```python
from build123d import *

# Parameters (mm, degrees)
F0_W     = 5
F0_H     = 40
F1_DEPTH = 5
F0_R     = 12.5
F2_DEPTH = 12
F0_R_2   = 5
F3_DEPTH = 5
F4_R     = 6
F5_DEPTH = 5
F6_R     = 6
F7_DEPTH = 5


with BuildPart() as f1:
    # F0 (on Top) → F1 (new body)
    with BuildSketch(Plane.XY):
        with Locations((37.5, 0)):
            Rectangle(F0_W, F0_H)
        with BuildLine():
            Line((0, -20), (35, -20))
            Line((35, -20), (35, 20))
            Line((35, 20), (0, 20))
            ThreePointArc((0, 20), (14.142136, 14.142136), (20, 0))
            ThreePointArc((20, 0), (14.142136, -14.142136), (0, -20))
        make_face()
        with BuildLine():
            Line((-35, -20), (0, -20))
            ThreePointArc((0, -20), (-20, 0), (0, 20))
            Line((0, 20), (-35, 20))
            Line((-35, 20), (-35, -20))
        make_face()
        with Locations((-37.5, 0)):
            Rectangle(F0_W, F0_H)
    extrude(amount=F1_DEPTH)

    # F0 (on Top) → F2 (join)
    with BuildSketch(Plane.XY):
        with BuildLine():
            ThreePointArc((0, 20), (-20, 0), (0, -20))
            ThreePointArc((0, -20), (14.142136, -14.142136), (20, 0))
            ThreePointArc((20, 0), (14.142136, 14.142136), (0, 20))
        make_face()
        Circle(F0_R, mode=Mode.SUBTRACT)
    extrude(amount=F2_DEPTH)

    # F0 (on Top) → F3 (join)
    with BuildSketch(Plane.XY):
        Circle(F0_R)
        Circle(F0_R_2, mode=Mode.SUBTRACT)
    extrude(amount=F3_DEPTH)

    # F4 (on face) → F5 (join)
    with BuildSketch(Plane(origin=(-40, 0, 0), x_dir=(0, -1, 0), z_dir=(-1, 0, 0))):
        with BuildLine():
            Line((20, 0), (-20, 0))
            Line((-20, 0), (-20, -37))
            ThreePointArc((-20, -37), (0, -57), (20, -37))
            Line((20, -37), (20, 0))
        make_face()
        with Locations((0, -37)):
            Circle(F4_R, mode=Mode.SUBTRACT)
    extrude(amount=-F5_DEPTH)

    # F6 (on face) → F7 (join)
    with BuildSketch(Plane.YZ.offset(40)):
        with BuildLine():
            Line((-20, 5), (-20, 0))
            Line((-20, 0), (-20, -37))
            ThreePointArc((-20, -37), (0, -57), (20, -37))
            Line((20, -37), (20, 0))
            Line((20, 0), (20, 5))
            Line((20, 5), (-20, 5))
        make_face()
        with Locations((0, -37)):
            Circle(F6_R, mode=Mode.SUBTRACT)
    extrude(amount=-F7_DEPTH)


solid = f1.part
```
CAD build for the part. Positions are in the model's coordinates, mm. A direction names the side the tool comes from. Coordinates: 2 decimals unless noted, no trailing zeros. Order: outer loops, then holes, each group sorted by start corner. A loop starts at its lowest first (then second) coordinate and runs counter-clockwise, first axis right, second up. Notation, with made-up numbers: (6, 58) -> (65, 58) arc R33 cw to (65, 89) -> close; hole circle Ø5 at (35.5, -16). An arc over 180 degrees is marked (long way). Use one line per item in the form item = value. Start each with the question number.
1) Band-saw the part on B-B on z = -36. Give the cut face in (x, y).
2) Band-saw the part on A-A on z = -24. Give the cut face in (x, y), then the cut area to 3 significant figures.
3) Drop flat-ended pins along their axis: pin 1 (20 mm diameter, centred on x = -9, y = -6, fed in from -Z); pin 2 (20 mm diameter, centred on x = 0, y = 0, fed in from +Z). Give the stop position or say it passes through.
4) Tool access for faces 1 (the cylindrical face through (11.923, 3.755, 8.451)), 2 (the flat face through (7, 0, 0)), 3 (the flat face through (29, 0, 5)): list every direction of +Z, -Z, +X, -X, +Y, -Y with a clear straight run to the whole face (end or side of a thin tool).
5) Drill centre lines: L1, parallel to X at y = 11, z = -2; L2, parallel to Y at x = 0, z = 7.5; L3, parallel to Y at x = 0, z = 2.5. Where is each one in solid material? Low to high. Write a range as [from, to].
6) Band-saw the part on C-C on x = -25. Give the cut face in (y, z), then the cut area to 3 significant figures.
7) Band-saw the part on D-D on y = -14.5. Give the cut face in (x, z).
8) Pull direction X, two halves, no side cores. Call faces 4 (the flat face through (40, 0, -26)), 5 (the flat face through (35, 0, -28)), 6 (the cylindrical face through (-37.535, 1.301, -42.857)): +X half, -X half, draft (parallel to the pull), parting line (faces both ways), or undercut.
Entries:
q1.outline = (-40, -20) -> (-35, -20) -> (-35, -5.92) -> (-40, -5.92) -> close; (-40, 5.92) -> (-35, 5.92) -> (-35, 20) -> (-40, 20) -> close; (35, -20) -> (40, -20) -> (40, -5.92) -> (35, -5.92) -> close; (35, 5.92) -> (40, 5.92) -> (40, 20) -> (35, 20) -> close
q2.outline = (-40, -20) -> (-35, -20) -> (-35, 20) -> (-40, 20) -> close; (35, -20) -> (40, -20) -> (40, 20) -> (35, 20) -> close
q2.area = 400 mm2
q3.pin_1 = 0
q3.pin_2 = 5
q4.face_1 = +Z
q4.face_2 = -Z, +Y, -Y
q4.face_3 = +Z, +X
q5.L1 = [-40, -35], [35, 40]
q5.L2 = [-20, -12.5], [12.5, 20]
q5.L3 = [-20, -5], [5, 20]
q6.outline = (-20, 0) -> (20, 0) -> (20, 5) -> (-20, 5) -> close
q6.area = 200 mm2
q7.outline = (-40, -50.77) -> (-35, -50.77) -> (-35, 0) -> (35, 0) -> (35, -50.77) -> (40, -50.77) -> (40, 5) -> (13.77, 5) -> (13.77, 12) -> (-13.77, 12) -> (-13.77, 5) -> (-40, 5) -> close
q8.face_4 = +X half
q8.face_5 = undercut
q8.face_6 = draft
